The listing builds one solid part. Answer for the finished solid, in the listing's coordinates (mm). Give positions to 0.01 mm unless a question says otherwise; leave off trailing zeros. Order: outer loops, then holes, each group sorted by start corner. A loop starts at its lowest first (then second) coordinate and runs counter-clockwise, first axis right, second up. Notation, with made-up numbers: (33, 45) - (42, 45) arc R15 cw to (42, 55) - close; hole circle Ø11 at (21, 61.25). An arc over 180 degrees is marked (long way). Answer as CSV lines item,"result". Start each with the question number.
1. Consider line 1 along Y through (x, z) = (139, 628); line 2 along Y through (x, z) = (45, 652). Determine where each line is inside the solid, lowest interval first. Write a range as [from, to].
2. Section C-C on z = 1020 is taken. Give the vertices of the cut face in (x, y), and give its area (3 significant figures).
3. Section A-A on z = -10 is taken. Give the vertices of the cut face in (x, y).
4. Section B-B on x = 179.5 is taken. Give the vertices of the cut face in (y, z).
5. Flat-ended cylindrical pins translate along their axes: pin 1 (2 mm diameter, centred on x = -70, z = 422.5, fed in from +Y); pin 2 (2 mm diameter, centred on x = 33, z = 879.5, fed in from -Y); pin 3 (7.5 mm diameter, centred on x = -254.5, y = -651, fed in from +Z); pin 4 (20.5 mm diameter, centred on y = -644, z = 317.5, fed in from +X). Find the tip coordinate at first contact, or state that the pin passes through.
from build123d import *

# Parameters (mm, degrees)
F0_W     = 609.6
F0_H     = 1651
F1_DEPTH = 609.6
F2_W     = 609.6
F2_H     = 1143
F2_H_2   = 495.3
F3_DEPTH = 25.4
F4_W     = 25.4
F4_H     = 381
F5_DEPTH = 25.4
F6_R     = 12.7


with BuildPart() as f1:
    # F0 (on Front) → F1 (new body)
    with BuildSketch(Plane.XZ):
        with Locations((-1.901709, 324.781201)):
            Rectangle(F0_W, F0_H)
    extrude(amount=F1_DEPTH)

    # F2 (on face) → F3 (join)
    with BuildSketch(Plane.XZ.offset(609.6)):
        with Locations((-1.901709, 70.781201)):
            Rectangle(F2_W, F2_H)
        with Locations((-1.901709, 902.631201)):
            Rectangle(F2_W, F2_H_2)
    extrude(amount=F3_DEPTH)

    # F4 (on face) → F5 (join)
    with BuildSketch(Plane.XZ.offset(635)):
        with Locations((-255.901709, 908.981201)):
            Rectangle(F4_W, F4_H)
        with Locations((-255.901709, 400.981201)):
            Rectangle(F4_W, F4_H)
    extrude(amount=F5_DEPTH)

    # F6
    f6_edges = [f1.edges().sort_by_distance(p)[0] for p in [
        (302.898291, -635, 902.631201),
        (302.898291, -635, 70.781201),
        (-306.701709, -635, 902.631201),
        (-306.701709, -635, 70.781201),
    ]]
    fillet(f6_edges, radius=F6_R)


solid = f1.part
Checks:
1,line 1,"y = [-635, 0]"
1,line 2,"y = [-609.6, 0]"
2,outline,"(-306.7, -622.3) arc R12.7 ccw to (-294, -635) - (-268.6, -635) - (-268.6, -660.4) - (-243.2, -660.4) - (-243.2, -635) - (290.2, -635) arc R12.7 ccw to (302.9, -622.3) - (302.9, 0) - (-306.7, 0) - close"
2,area,"388,000 mm²"
3,outline,"(-306.7, -622.3) arc R12.7 ccw to (-294, -635) - (290.2, -635) arc R12.7 ccw to (302.9, -622.3) - (302.9, 0) - (-306.7, 0) - close"
4,outline,"(-635, -500.72) - (0, -500.72) - (0, 1150.28) - (-635, 1150.28) - (-635, 654.98) - (-609.6, 654.98) - (-609.6, 642.28) - (-635, 642.28) - close"
5,pin 1,"stops at y = 0"
5,pin 2,"stops at y = -635"
5,pin 3,"stops at z = 1099.48"
5,pin 4,"stops at x = 295.69"
